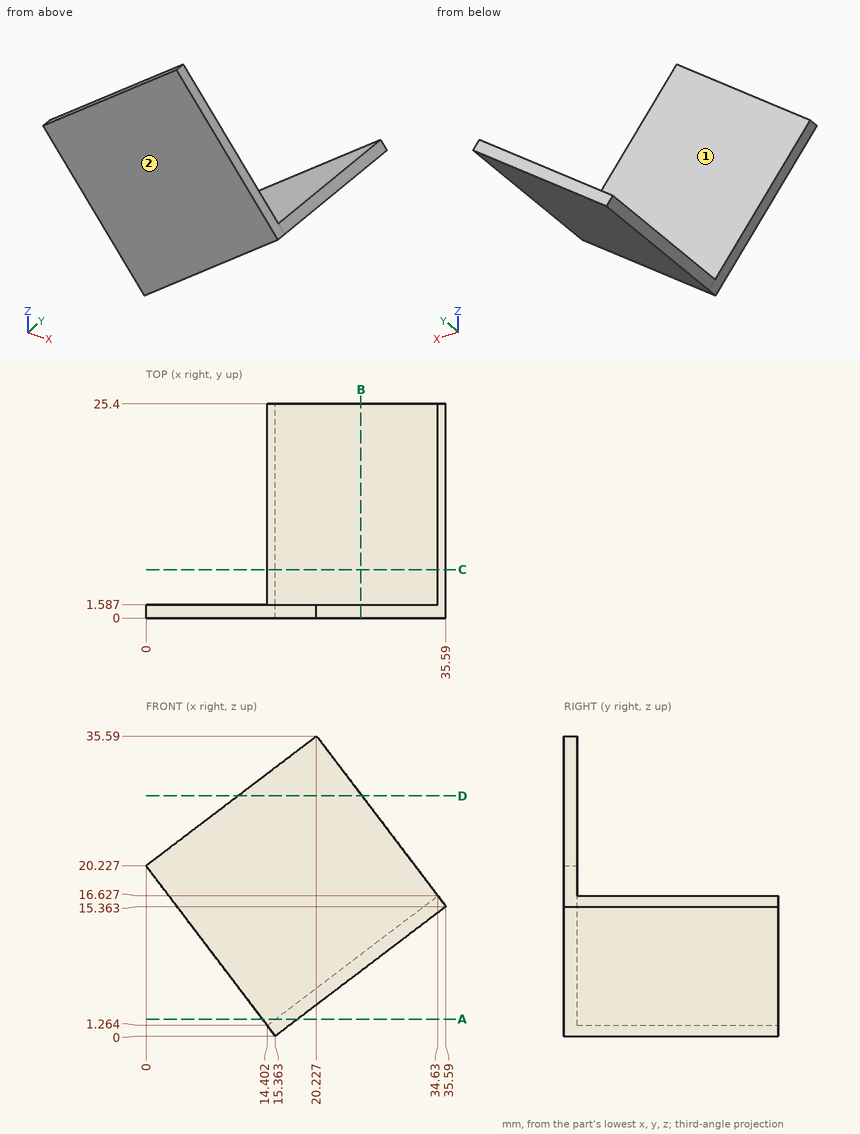
Job drawing, mm, ordinate dimensions from the low corner. One solid piece. A direction names the side the tool comes from. Coordinates: 2 decimals unless noted, no trailing zeros. Order: outer loops, then holes, each group sorted by start corner. A loop starts at its lowest first (then second) coordinate and runs counter-clockwise, first axis right, second up. Notation, with made-up numbers: (-33, 74) - (2, 74) arc R5 ccw to (2, 83) - close; hole circle Ø2 at (31, 9). An arc over 180 degrees is marked (long way). Write each question's results on one line, items separated by ' | '. Start each with the question number.
Item 1: Band-saw the part on C-C on y = 5.75. Write the cut outline in (x, z) (1 decimal).
Item 2: Wall check: probe 1 along Y at (x, z) = (17, 25.5); probe 2 along Z at (x, y) = (21, 17) (1 decimal); probe 3 along X at (y, z) = (17.25, 3.5) (1 decimal). Give the ranges that are in metal, low to high. Write a range as [from, to].
Item 3: Band-saw the part on B-B on x = 25.5. Write the cut outline in (y, z).
Item 4: Flat gauge pins, fed straight in: pin 1 (8 mm diameter, centred on x = 6, y = 2.5, fed in from +Z); pin 2 (1 mm diameter, centred on y = 11.5, z = 8, fed in from -X) (1 decimal); pin 3 (6 mm diameter, centred on x = 23, z = 25.5, fed in from +Y). Where does each tip first touch, or does it go through?
Item 5: Band-saw the part on A-A on z = 2. Write the cut outline in (x, y) (1 decimal).
Item 6: Band-saw the part on D-D on z = 28.5. Write the cut outline in (x, y).
Item 7: Tool access for the marked faces 1 and 2: list every direction of +Z, -Z, +X, -X, +Y, -Y with a clear straight run to the whole face (end or side of a thin tool).
Numbers:
1) outline: (14.4, 1.3) - (15.4, 0) - (35.6, 15.4) - (34.6, 16.6) - close
2) probe 1: [0, 1.59] | probe 2: [4.3, 6.3] | probe 3: [17.3, 20]
3) outline: (0, 7.7) - (25.4, 7.7) - (25.4, 9.69) - (1.59, 9.69) - (1.59, 28.65) - (0, 28.65) - close
4) pin 1: z = 27.74 | pin 2: x = 22.6 | pin 3: y = 1.59
5) outline: (13.8, 0) - (18, 0) - (18, 25.4) - (15.4, 25.4) - (15.4, 1.6) - (13.8, 1.6) - close
6) outline: (10.89, 0) - (25.61, 0) - (25.61, 1.59) - (10.89, 1.59) - close
7) face 1: +Z, -X, +Y | face 2: +Z, -Z, +X, -X, -Y
